Geometry: final body of the model. Coordinates: model frame, mm. A direction names the side the tool comes from. Round coordinates to 2 decimals unless told otherwise and drop trailing zeros. Loops run counter-clockwise (first coordinate to the right, second up) from the corner with the lowest first, then second, coordinate; pieces in that order, holes last. Notation, with made-up numbers: (14, -22) -> (50, -22) arc R27 cw to (50, 16) -> close; hole circle Ø5 at (16.25, 74.25). An arc over 180 degrees is marked (long way). Answer in a Markdown table with one row per item.
```python
from build123d import *

# Parameters (mm, degrees)
F0_W     = 2000
F0_H     = 1000
F0_W_2   = 100
F0_H_2   = 100
F1_DEPTH = 25
F2_DEPTH = 725
F3_R     = 33.258786
F3_R_2   = 35.777632
F3_R_3   = 37.427227
F4_DEPTH = 950.001
F5_R     = 25
F6_DEPTH = 950.001


with BuildPart() as f1:
    # F0 (on Front) → F1 (new body)
    with BuildSketch(Plane.XZ):
        with Locations((-6.459419, 11.359975)):
            Rectangle(F0_W, F0_H)
        with Locations((-906.459419, -388.640025)):
            Rectangle(F0_W_2, F0_H_2, mode=Mode.SUBTRACT)
        with Locations((893.540581, -388.640025)):
            Rectangle(F0_W_2, F0_H_2, mode=Mode.SUBTRACT)
        with Locations((-906.459419, 411.359975)):
            Rectangle(F0_W_2, F0_H_2, mode=Mode.SUBTRACT)
        with Locations((893.540581, 411.359975)):
            Rectangle(F0_W_2, F0_H_2, mode=Mode.SUBTRACT)
    extrude(amount=F1_DEPTH)

    # F0 (on Front) → F2 (join)
    with BuildSketch(Plane.XZ):
        with Locations((893.540581, -388.640025)):
            Rectangle(F0_W_2, F0_H_2)
        with Locations((-906.459419, -388.640025)):
            Rectangle(F0_W_2, F0_H_2)
        with Locations((-906.459419, 411.359975)):
            Rectangle(F0_W_2, F0_H_2)
        with Locations((893.540581, 411.359975)):
            Rectangle(F0_W_2, F0_H_2)
    extrude(amount=F2_DEPTH)

    # F3 (on face) → F4 (cut, through all)
    with BuildSketch(Plane(origin=(0, 0, -438.640025), x_dir=(1, 0, 0), z_dir=(0, 0, -1))):
        with Locations((-906.459419, 125)):
            Circle(F3_R)
        with Locations((-906.459419, 325)):
            Circle(F3_R_2)
        with Locations((-906.459419, 525)):
            Circle(F3_R_3)
    extrude(amount=-F4_DEPTH, mode=Mode.SUBTRACT)

    # F5 (on face) → F6 (cut, through all)
    with BuildSketch(Plane.XY.offset(461.359975)):
        with Locations((893.540581, -525)):
            Circle(F5_R)
        with Locations((893.540581, -325)):
            Circle(F5_R)
        with Locations((893.540581, -125)):
            Circle(F5_R)
    extrude(amount=-F6_DEPTH, mode=Mode.SUBTRACT)


solid = f1.part
```
Item 1: Section query C-C, the plane y = -525. State how many separate pieces and enclosed holes the cut face has, and give its area (3 significant figures).
Ans:
| item | result |
|---|---|
| separate pieces | 8 |
| enclosed holes | 0 |
| area | 15,000 mm2 |
Item 2: Section query B-B, the plane z = 430. Output: boundary loops of the cut face in (x, y).
Ans:
| item | result |
|---|---|
| outline | (-1006.46, -25) -> (-956.46, -25) -> (-956.46, -725) -> (-856.46, -725) -> (-856.46, -25) -> (843.54, -25) -> (843.54, -725) -> (943.54, -725) -> (943.54, -25) -> (993.54, -25) -> (993.54, 0) -> (-1006.46, 0) -> close; hole circle Ø74.85 at (-906.46, -525); hole circle Ø71.56 at (-906.46, -325); hole circle Ø66.52 at (-906.46, -125); hole circle Ø50 at (893.54, -525); hole circle Ø50 at (893.54, -325); hole circle Ø50 at (893.54, -125) |
Item 3: Section query A-A, the plane y = -44. Output: boundary loops of the cut face in (x, z).
Ans:
| item | result |
|---|---|
| outline | (-956.46, -438.64) -> (-856.46, -438.64) -> (-856.46, -338.64) -> (-956.46, -338.64) -> close; (-956.46, 361.36) -> (-856.46, 361.36) -> (-856.46, 461.36) -> (-956.46, 461.36) -> close; (843.54, -438.64) -> (943.54, -438.64) -> (943.54, -338.64) -> (843.54, -338.64) -> close; (843.54, 361.36) -> (943.54, 361.36) -> (943.54, 461.36) -> (843.54, 461.36) -> close |
Item 4: Section query D-D, the plane x = -255. Output: boundary loops of the cut face in (y, z).
Ans:
| item | result |
|---|---|
| outline | (-25, -488.64) -> (0, -488.64) -> (0, 511.36) -> (-25, 511.36) -> close |
Item 5: Ray query, L1, parallel to X at y = -292, z = -392; L2, parallel to Y at x = 881, z = 374; L3, parallel to Z at x = -920, y = -42. Return the intervals inside material, ascending.
Ans:
| item | result |
|---|---|
| L1 | -956.46 to -920.28, -892.64 to -856.46, 843.54 to 943.54 |
| L2 | -725 to -546.63, -503.37 to -346.63, -303.37 to -146.63, -103.37 to 0 |
| L3 | -438.64 to -338.64, 361.36 to 461.36 |
Item 6: First-contact query: P1, Ø4, axis at x = 348, z = 33, coming from the -Y side. Flat tip, straight axial feed; report the tip coordinate or a pass-through.
Ans:
| item | result |
|---|---|
| P1 | y = -25 |
Item 7: Mould query, pull axis Z, two halves, no side actions, for faces 6 (the flat face through (843.541, -370, -389)), 7 (the flat face through (-907, -370, 361.36)), 8 (the flat face through (-907, -370, -338.64)), 9 (the flat face through (893, -370, -438.64)). Classes: released by +Z, released by -Z, zero draft, split by the parting line, or undercut.
Ans:
| item | result |
|---|---|
| face 6 | zero draft |
| face 7 | undercut |
| face 8 | undercut |
| face 9 | released by -Z |
Item 8: Set-up query: faces 1 (the flat face through (893, -370, 461.36)), 2 (the flat face through (-956.459, -370, 411)), 3 (the flat face through (843.541, -370, 411)), 4 (the cylindrical face through (875.115, -508.104, -387.94)), 5 (the flat face through (943.541, -370, 411)). Return all of +Z, -Z, +X, -X, +Y, -Y with unobstructed straight access to the full face (end or side cutting, diameter ignored); none if empty.
Ans:
| item | result |
|---|---|
| face 1 | +Z, +X, -X, -Y |
| face 2 | +Z, -Z, -X, -Y |
| face 3 | +Z, -Z, -Y |
| face 4 | +Z, -Z |
| face 5 | +Z, -Z, +X, -Y |
